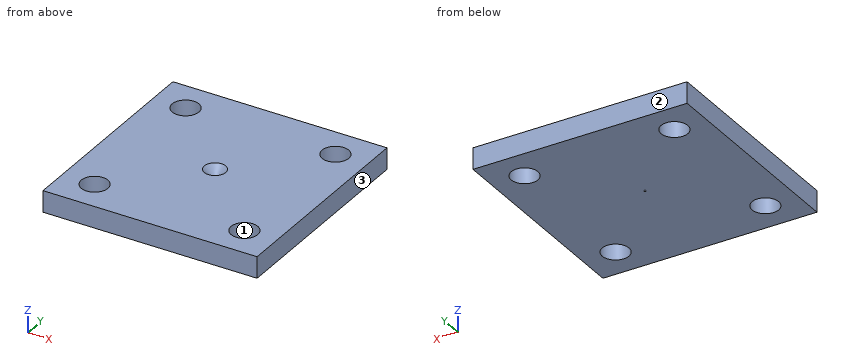
from build123d import *

# Parameters (mm, degrees)
F0_W     = 20
F0_H     = 20
F1_DEPTH = 1
F2_R     = 1
F3_R     = 0.1
F6_W     = 20
F6_H     = 20
F6_R     = 0.1
F7_DEPTH = 1
F8_D     = 2.5


with BuildPart() as f1:
    # F0 (on Top) → F1 (new body)
    with BuildSketch(Plane.XY):
        Rectangle(F0_W, F0_H)
    extrude(amount=-F1_DEPTH)

    # F2 (on face) → F4 section 0
    with BuildSketch(Plane.XY):
        Circle(F2_R)
    # F3 (on face) → F4 section 1
    with BuildSketch(Plane(origin=(0, 0, -1), x_dir=(1, 0, 0), z_dir=(0, 0, -1))):
        Circle(F3_R)
    loft(mode=Mode.SUBTRACT)

    # F6 (on face) → F7 (join)
    with BuildSketch(Plane(origin=(0, 0, -1), x_dir=(1, 0, 0), z_dir=(0, 0, -1))):
        Rectangle(F6_W, F6_H)
        Circle(F6_R, mode=Mode.SUBTRACT)
    extrude(amount=F7_DEPTH)

    # F8 (through all)
    with Locations(Plane.XY):
        with Locations((-7, -7), (7, -7), (7, 7), (-7, 7)):
            Hole(F8_D / 2)


solid = f1.part
Could you check a few things on this model? Use its own coordinates, in mm. Face numbers are marked on the shaded views. Give positions to 0.01 mm unless a question says otherwise; leave off trailing zeros. Order: outer loops, then holes, each group sorted by start corner. A loop starts at its lowest first (then second) coordinate and runs counter-clockwise, first axis right, second up. Notation, with made-up numbers: M -31.5,40.25 L 27.5,40.25 A20 ccw 27.5,74.25 Z; hole C 87.5,-19 d1. An arc over 180 degrees is marked long. One line per question, with ' | ' between items.
1. We'd pull the mould along X, two halves only. Please class the marked faces 1, 2 and 3: +X half, -X half, draft (parallel to the pull), parting line (faces both ways), or undercut.
Results:
face 1: undercut | face 2: draft | face 3: +X half
2. I want a section at A-A (x = 7). List the corners of the cut face in (y, z) for me.
Results:
outline: M -10,-2 L -8.25,-2 L -8.25,0 L -10,0 Z; M -5.75,-2 L 5.75,-2 L 5.75,0 L -5.75,0 Z; M 8.25,-2 L 10,-2 L 10,0 L 8.25,0 Z
3. If I drill on line 1 (Y direction, x = 7, z = -0.95); line 2 (Y direction, x = 0, z = -1.4); line 3 (X direction, y = 6, z = -0.95), over which ranges is the centre line in solid material (lowest first)?
Results:
line 1: -10 to -8.25, -5.75 to 5.75, 8.25 to 10 | line 2: -10 to -0.1, 0.1 to 10 | line 3: -10 to -7.75, -6.25 to 6.25, 7.75 to 10
4. I'm going to push a flat-ended pin straight in: pin 1 (10 mm diameter, centred on x = -7.5, y = 6.5, fed in from +Z). Where does the tip first touch, or does it pass through?
Results:
pin 1: z = 0
5. I want a section at B-B (y = 6.25). List the corners of the cut face in (x, z) for me.
Results:
outline: M -10,-2 L -8,-2 L -8,0 L -10,0 Z; M -6,-2 L 6,-2 L 6,0 L -6,0 Z; M 8,-2 L 10,-2 L 10,0 L 8,0 Z
